Could you check a few things on this model? Use its own coordinates, in mm. A direction names the side the tool comes from. Round coordinates to 2 decimals unless told otherwise and drop trailing zeros. Order: outer loops, then holes, each group sorted by start corner. A loop starts at its lowest first (then second) coordinate and runs counter-clockwise, first axis right, second up. Notation, with made-up numbers: (-23.5, -31.5) -> (-12.5, -31.5) arc R22 ccw to (-12.5, -3.5) -> close; hole circle Ø11 at (33.25, -32). An arc over 180 degrees is marked (long way). One line per question, with ' | ' between items.
```python
from build123d import *

# Parameters (mm, degrees)
ESQUISSE1_R        = 45
ESQUISSE1_R_2      = 2.25
BOSS_EXTRU_1_DEPTH = 7
BOSS_EXTRU_2_DEPTH = 3
BOSS_EXTRU_3_START = 2.5
BOSS_EXTRU_3_DEPTH = 2.5
CONG_1_R           = 5


with BuildPart() as part:
    # Esquisse1 → Boss.-Extru.1 (new body)
    with BuildSketch(Plane.XY):
        with BuildLine():
            Line((20, 0), (88, 0))
            ThreePointArc((88, 0), (102.142135624, -5.857864376), (108, -20))
            Line((108, -20), (108, -88))
            ThreePointArc((108, -88), (102.142135624, -102.142135624), (88, -108))
            Line((88, -108), (20, -108))
            ThreePointArc((20, -108), (5.857864376, -102.142135624), (0, -88))
            Line((0, -88), (0, -20))
            ThreePointArc((0, -20), (5.857864376, -5.857864376), (20, 0))
        make_face()
        with Locations((54, -54)):
            Circle(ESQUISSE1_R, mode=Mode.SUBTRACT)
        with Locations((14, -14)):
            Circle(ESQUISSE1_R_2, mode=Mode.SUBTRACT)
        with Locations((94, -14)):
            Circle(ESQUISSE1_R_2, mode=Mode.SUBTRACT)
        with Locations((94, -94)):
            Circle(ESQUISSE1_R_2, mode=Mode.SUBTRACT)
        with Locations((14, -94)):
            Circle(ESQUISSE1_R_2, mode=Mode.SUBTRACT)
    extrude(amount=BOSS_EXTRU_1_DEPTH)

    # Esquisse2 → Boss.-Extru.2 (add)
    with BuildSketch(Plane.XY.offset(7)):
        with BuildLine():
            Line((20, 0), (88, 0))
            ThreePointArc((88, 0), (102.142135624, -5.857864376), (108, -20))
            Line((108, -20), (108, -88))
            ThreePointArc((108, -88), (102.142135624, -102.142135624), (88, -108))
            Line((88, -108), (20, -108))
            ThreePointArc((20, -108), (5.857864376, -102.142135624), (0, -88))
            Line((0, -88), (0, -20))
            ThreePointArc((0, -20), (5.857864376, -5.857864376), (20, 0))
        make_face()
        with BuildLine():
            Line((22.5, -2.5), (85.5, -2.5))
            ThreePointArc((85.5, -2.5), (99.642135624, -8.357864376), (105.5, -22.5))
            Line((105.5, -22.5), (105.5, -85.5))
            ThreePointArc((105.5, -85.5), (99.642135624, -99.642135624), (85.5, -105.5))
            Line((85.5, -105.5), (22.5, -105.5))
            ThreePointArc((22.5, -105.5), (8.357864376, -99.642135624), (2.5, -85.5))
            Line((2.5, -85.5), (2.5, -22.5))
            ThreePointArc((2.5, -22.5), (8.357864376, -8.357864376), (22.5, -2.5))
        make_face(mode=Mode.SUBTRACT)
    extrude(amount=BOSS_EXTRU_2_DEPTH)

    # Esquisse3 → Boss.-Extru.3 (add)
    with BuildSketch(Plane(origin=(0, 0, 0), x_dir=(-1, 0, 0), z_dir=(0, 0, -1)).offset(BOSS_EXTRU_3_START)):
        with BuildLine():
            Line((-20, 0), (-88, 0))
            ThreePointArc((-88, 0), (-102.142135624, -5.857864376), (-108, -20))
            Line((-108, -20), (-108, -88))
            ThreePointArc((-108, -88), (-102.142135624, -102.142135624), (-88, -108))
            Line((-88, -108), (-20, -108))
            ThreePointArc((-20, -108), (-5.857864376, -102.142135624), (0, -88))
            Line((0, -88), (0, -20))
            ThreePointArc((0, -20), (-5.857864376, -5.857864376), (-20, 0))
        make_face()
        with BuildLine():
            Line((-84, -104), (-24, -104))
            ThreePointArc((-24, -104), (-9.857864376, -98.142135624), (-4, -84))
            Line((-4, -84), (-4, -24))
            ThreePointArc((-4, -24), (-9.857864376, -9.857864376), (-24, -4))
            Line((-24, -4), (-84, -4))
            ThreePointArc((-84, -4), (-98.142135624, -9.857864376), (-104, -24))
            Line((-104, -24), (-104, -84))
            ThreePointArc((-104, -84), (-98.142135624, -98.142135624), (-84, -104))
        make_face(mode=Mode.SUBTRACT)
    extrude(amount=-BOSS_EXTRU_3_DEPTH)

    # Congé1
    # the kernel refuses this fillet: 5 mm, written as the material it takes off along each edge
    with BuildSketch(Plane(origin=(88, -88, -2.5), x_dir=(1, 0, 0), z_dir=(0, 1, 0))) as cong_1_piece_1:
        with BuildLine():
            CenterArc((20 - CONG_1_R, -CONG_1_R), CONG_1_R, 0, 90)
            Line((20 - CONG_1_R, 0), (20, 0))
            Line((20, 0), (20, -CONG_1_R))
        make_face()
    revolve(axis=Axis((88, -88, -2.5), (0, 0, -1)), revolution_arc=90, mode=Mode.SUBTRACT)
    with BuildSketch(Plane(origin=(88, -20, -2.5), x_dir=(0, 1, 0), z_dir=(-1, 0, 0))) as cong_1_piece_2:
        with BuildLine():
            CenterArc((20 - CONG_1_R, -CONG_1_R), CONG_1_R, 0, 90)
            Line((20 - CONG_1_R, 0), (20, 0))
            Line((20, 0), (20, -CONG_1_R))
        make_face()
    revolve(axis=Axis((88, -20, -2.5), (0, 0, -1)), revolution_arc=90, mode=Mode.SUBTRACT)
    with BuildSketch(Plane(origin=(20, -20, -2.5), x_dir=(-1, 0, 0), z_dir=(0, -1, 0))) as cong_1_piece_3:
        with BuildLine():
            CenterArc((20 - CONG_1_R, -CONG_1_R), CONG_1_R, 0, 90)
            Line((20, -CONG_1_R), (20, 0))
            Line((20, 0), (20 - CONG_1_R, 0))
        make_face()
    revolve(axis=Axis((20, -20, -2.5), (0, 0, -1)), revolution_arc=90, mode=Mode.SUBTRACT)
    with BuildSketch(Plane(origin=(20, -88, -2.5), x_dir=(0, -1, 0), z_dir=(1, 0, 0))) as cong_1_piece_4:
        with BuildLine():
            CenterArc((20 - CONG_1_R, -CONG_1_R), CONG_1_R, 0, 90)
            Line((20 - CONG_1_R, 0), (20, 0))
            Line((20, 0), (20, -CONG_1_R))
        make_face()
    revolve(axis=Axis((20, -88, -2.5), (0, 0, -1)), revolution_arc=90, mode=Mode.SUBTRACT)
    with BuildSketch(Plane(origin=(88, -108, -2.5), x_dir=(0, 0, 1), z_dir=(-1, 0, 0)), Plane(origin=(0, -88, -2.5), x_dir=(0, 0, 1), z_dir=(0, 1, 0)), Plane(origin=(20, 0, -2.5), x_dir=(0, 0, 1), z_dir=(1, 0, 0)), Plane(origin=(108, -20, -2.5), x_dir=(0, 0, 1), z_dir=(0, -1, 0))) as cong_1_piece_5:
        with BuildLine():
            CenterArc((CONG_1_R, CONG_1_R), CONG_1_R, 180, 90)
            Line((0, CONG_1_R), (0, 0))
            Line((0, 0), (CONG_1_R, 0))
        make_face()
    extrude(amount=68, mode=Mode.SUBTRACT)


solid = part.part
```
1. I want a section at A-A on y = -54. List the corners of the cut face in (x, z) for me.
From the geometry:
outline: (0, 2.5) arc R5 ccw to (4, -2.4) -> (4, 0) -> (9, 0) -> (9, 7) -> (2.5, 7) -> (2.5, 10) -> (0, 10) -> close; (99, 0) -> (104, 0) -> (104, -2.4) arc R5 ccw to (108, 2.5) -> (108, 10) -> (105.5, 10) -> (105.5, 7) -> (99, 7) -> close
2. I want a section at D-D on x = 14. Count the separate pieces of the cut face and the enclosed holes in it, and give its area (3 significant figures).
From the geometry:
separate pieces: 4 | enclosed holes: 0 | area: 430 mm²
3. I want a section at B-B on z = 5.25. List the corners of the cut face in (x, y) for me.
From the geometry:
outline: (0, -88) arc R20 ccw to (20, -108) -> (88, -108) arc R20 ccw to (108, -88) -> (108, -20) arc R20 ccw to (88, 0) -> (20, 0) arc R20 ccw to (0, -20) -> close; hole circle Ø90 at (54, -54); hole circle Ø4.5 at (14, -94); hole circle Ø4.5 at (14, -14); hole circle Ø4.5 at (94, -94); hole circle Ø4.5 at (94, -14)
4. I want a section at C-C on x = 54. List the corners of the cut face in (y, z) for me.
From the geometry:
outline: (-108, 2.5) arc R5 ccw to (-104, -2.4) -> (-104, 0) -> (-99, 0) -> (-99, 7) -> (-105.5, 7) -> (-105.5, 10) -> (-108, 10) -> close; (-9, 0) -> (-4, 0) -> (-4, -2.4) arc R5 ccw to (0, 2.5) -> (0, 10) -> (-2.5, 10) -> (-2.5, 7) -> (-9, 7) -> close
5. If we mould it in two halves opening along X, with no side actions, what happens to faces 4 (the face through (105.5, -54, 8)), 5 (the face through (18, -81, 3)), 6 (the face through (5.703, -6.014, 6.198)), 7 (the face through (54, 0, 6))? For each: pulls with the +X half, pulls with the -X half, needs draft (parallel to the pull), parting line crosses it, or undercut.
From the geometry:
face 4: undercut | face 5: undercut | face 6: pulls with the -X half | face 7: needs draft
6. I need wall thicknesses on probe 1 along Y at (x, z) = (54, 2.5); probe 2 along Y at (x, z) = (14, 3); probe 3 along X at (y, z) = (-34.5, 8.5). Which ranges of each line are inside material? Lowest first, please.
From the geometry:
probe 1: y = -108 to -99, -9 to 0 | probe 2: y = -107.08 to -96.25, -91.75 to -74.62, -33.38 to -16.25, -11.75 to -0.92 | probe 3: x = 0 to 2.5, 105.5 to 108
7. I'm going to push flat-ended pins straight in: pin 1 (5 mm diameter, centred on x = 94, y = -14, fed in from +Z); pin 2 (6 mm diameter, centred on x = 94, y = -94, fed in from -Z); pin 3 (2.5 mm diameter, centred on y = -61.5, z = -1, fed in from -X); pin 4 (3.5 mm diameter, centred on x = 14, y = -94, fed in from +Z). Where does each tip first touch, or does it pass through?
From the geometry:
pin 1: stops at z = 7 | pin 2: stops at z = 0 | pin 3: stops at x = 0.53 | pin 4: passes through
8. On a 3-axis mill with a long thin cutter (end or side, diameter ignored), from which of +Z, -Z, +X, -X, +Y, -Y can I reach the whole of each face in a straight line? I mean faces 1 (the face through (0, -54, 6)), 2 (the face through (10.014, -98.297, -1.268)), 3 (the face through (99.797, -99.486, 8.479)). Say none if no direction works.
From the geometry:
face 1: +Z, -Z, -X, +Y, -Y | face 2: -Z | face 3: +Z
